Source: CAD feature listing. Evaluate the final solid. Frame: model axes, mm. Face numbers are marked on the shaded views. A direction names the side the tool comes from. Give positions to 0.01 mm unless a question says otherwise; leave off trailing zeros. Write each loop counter-clockwise with the first axis right and the second up, starting at its lowest first coordinate (ties: lowest second). Pieces come first, ordered by that corner, then holes. Notation, with made-up numbers: (-34, -3) -> (-14, -3) arc R21 ccw to (-14, 17) -> close; hole circle Ø7 at (87, 83.5). An arc over 180 degrees is marked (long way). Answer as a JSON object with one key per item and string values. Group by question number.
Item 1: Section query D-D on x = 15. Return the cut outline in (y, z), plus the area to 3 significant figures.
Item 2: Section query A-A on y = 0. Return the cut outline in (x, z), plus the area to 3 significant figures.
Item 3: Ray query, probe 1 along Z at (x, y) = (-4, 7.5); probe 2 along Z at (x, y) = (0, -8.5); probe 3 along X at (y, z) = (-13.5, -5). Return the intervals inside material, ascending. Write a range as from..to.
Item 4: Section query B-B on x = -12. Return the cut outline in (y, z), plus the area to 3 significant figures.
Item 5: First-contact query: pin 1 Ø11 at (x, y) = (6.5, 0.5) entering from -Z; pin 2 Ø5 at (y, z) = (-2, -37) entering from -X; pin 3 Ø10 at (y, z) = (12, -12) entering from +X; pin 4 Ø3 at (x, z) = (-2.5, -41.5) entering from +Y. Flat tips, straight axial feed; report the tip coordinate or a pass-through.
Item 6: Access query for the marked faces 1, 2 and 3. Directions: +Z, -Z, +X, -X, +Y, -Y. A direction counts if a zero-diameter tool reaches every point of the face in a straight line with its end or side. Return the directions, or none.
Item 7: Section query C-C on z = -56. Return the cut outline in (x, y).
from build123d import *

# Parameters (mm, degrees)
SKETCH1_W           = 18.5
SKETCH1_H           = 25
SKETCH2_R           = 14
BOSS_EXTRUDE1_DEPTH = 42
FILLET1_R           = 1


with BuildPart() as part:
    # Sketch1 → Revolve1 (revolve)
    with BuildSketch(Plane.XZ, mode=Mode.PRIVATE) as revolve1_sk:
        with Locations((9.25, -12.5)):
            Rectangle(SKETCH1_W, SKETCH1_H)
    revolve(revolve1_sk.sketch.rotate(Axis((0, 0, 0), (0, 0, -1)), 180), axis=Axis((0, 0, 0), (0, 0, -1)))

    # Sketch2 → Boss-Extrude1 (add)
    with BuildSketch(Plane.XY):
        with Locations(Location((0, 0, 0), (0, 0, 180))):
            Circle(SKETCH2_R)
    extrude(amount=BOSS_EXTRUDE1_DEPTH)

    # Sketch3 → Revolve2 (revolve)
    with BuildSketch(Plane.XZ.offset(-7.419045711), mode=Mode.PRIVATE) as revolve2_sk:
        Polygon((5.757740364, -25), (-0.242259636, -25), (-0.242259636, -64.5), (2.757740364, -64.5), (2.757740364, -34.5), (5.757740364, -34.5), align=None)
    revolve(revolve2_sk.sketch.rotate(Axis((-0.242259636, 7.419045711, -25), (0, 0, -1)), 180), axis=Axis((-0.242259636, 7.419045711, -25), (0, 0, -1)))

    # Fillet1
    fillet1_edges = [part.edges().sort_by_distance(p)[0] for p in [
        (5.757740364, 7.419045711, -34.5),
    ]]
    fillet(fillet1_edges, radius=FILLET1_R)


solid = part.part
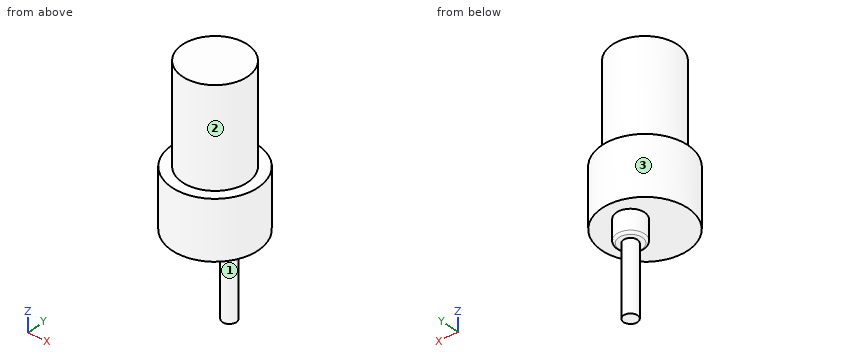
Worked answers:
{
 "1": {"outline": "(-10.83, -25) -> (10.83, -25) -> (10.83, 0) -> (-10.83, 0) -> close", "area": "541 mm^2"},
 "2": {"outline": "(-18.5, -25) -> (18.5, -25) -> (18.5, 0) -> (14, 0) -> (14, 42) -> (-14, 42) -> (-14, 0) -> (-18.5, 0) -> close", "area": "2,100 mm^2"},
 "3": {"probe 1": "-34.5..42", "probe 2": "-25..42", "probe 3": "-12.65..12.65"},
 "4": {"outline": "(-14.08, -25) -> (14.08, -25) -> (14.08, 0) -> (7.21, 0) -> (7.21, 42) -> (-7.21, 42) -> (-7.21, 0) -> (-14.08, 0) -> close", "area": "1,310 mm^2"},
 "5": {"pin 1": "z = -34.5", "pin 2": "through", "pin 3": "x = 17.12", "pin 4": "y = 10.32"},
 "6": {"face 1": "-Z", "face 2": "+Z", "face 3": "+Z, -Z"},
 "7": {"outline": "circle Ø6 at (-0.24, 7.42)"}
}
